Work out the finished part from the listing and answer in its coordinate system (mm). Face numbers are marked on the shaded views. A direction names the side the tool comes from. Round coordinates to 2 decimals unless told otherwise and drop trailing zeros. Loops run counter-clockwise (first coordinate to the right, second up) from the corner with the lowest first, then second, coordinate; pieces in that order, holes last. Notation, with made-up numbers: (82.25, 8) -> (100.25, 8) arc R19 ccw to (100.25, 40) -> close; hole circle Ø11 at (-38.75, 35). An arc over 180 degrees is marked (long way). Write item = value, one per line. Start each with the question number.
```python
from build123d import *

# Parameters (mm, degrees)
SKETCH_W        = 96
SKETCH_H        = 70
PAD_DEPTH       = 22.8
SKETCH001_W     = 92.6
SKETCH001_H     = 67
POCKET_DEPTH    = 21.8
SKETCH002_W     = 6.6
SKETCH002_H     = 6.6
PAD001_DEPTH    = 17.2
SKETCH003_W     = 61
SKETCH003_H     = 46
POCKET001_DEPTH = 1.001
SKETCH004_R     = 1.35
POCKET002_DEPTH = 10
SKETCH005_R     = 1.35
POCKET003_DEPTH = 10
SKETCH006_R     = 1.35
POCKET004_DEPTH = 10
SKETCH007_R     = 1.35
POCKET005_DEPTH = 10
POCKET006_DEPTH = 1.701
SKETCH009_W     = 7
SKETCH009_H     = 6.3
PAD002_DEPTH    = 12.2
SKETCH010_R     = 2.2
POCKET007_DEPTH = 13.201
SKETCH011_R     = 2.2
POCKET008_DEPTH = 13.201
SKETCH012_R     = 2.2
POCKET009_DEPTH = 13.201
SKETCH013_R     = 2.2
POCKET010_DEPTH = 13.201
SKETCH014_W     = 9.6
SKETCH014_H     = 15.6
POCKET011_DEPTH = 1.501
SKETCH015_W     = 8.6
SKETCH015_H     = 3.6
POCKET012_DEPTH = 1.501
FILLET_R        = 1
FILLET001_R     = 1
CHAMFER_SIZE    = 0.2
FILLET002_R     = 1
FILLET003_R     = 1


with BuildPart() as part:
    # Sketch → Pad (new body)
    with BuildSketch(Plane.XY):
        Rectangle(SKETCH_W, SKETCH_H)
    extrude(amount=PAD_DEPTH)

    # Sketch001 (on Face6 of Pad) → Pocket (cut)
    with BuildSketch(Plane.XY.offset(22.8)):
        Rectangle(SKETCH001_W, SKETCH001_H)
    extrude(amount=-POCKET_DEPTH, mode=Mode.SUBTRACT)

    # Sketch002 (on Face11 of Pocket) → Pad001 (join)
    with BuildSketch(Plane.XY.offset(1)):
        with Locations((-43, 30.2)):
            Rectangle(SKETCH002_W, SKETCH002_H)
        with Locations((43, 30.2)):
            Rectangle(SKETCH002_W, SKETCH002_H)
        with Locations((43, -30.2)):
            Rectangle(SKETCH002_W, SKETCH002_H)
        with Locations((-43, -30.2)):
            Rectangle(SKETCH002_W, SKETCH002_H)
    extrude(amount=PAD001_DEPTH)

    # Sketch003 (on Face13 of Pad001) → Pocket001 (cut, through all)
    with BuildSketch(Plane.XY.offset(1)):
        with Locations((0.3, 0.2)):
            Rectangle(SKETCH003_W, SKETCH003_H)
    extrude(amount=-POCKET001_DEPTH, mode=Mode.SUBTRACT)

    # Sketch004 (on Face19 of Pocket001) → Pocket002 (cut)
    with BuildSketch(Plane.XY.offset(18.2)):
        with Locations((-43, 30.2)):
            Circle(SKETCH004_R)
    extrude(amount=-POCKET002_DEPTH, mode=Mode.SUBTRACT)

    # Sketch005 (on Face16 of Pocket002) → Pocket003 (cut)
    with BuildSketch(Plane.XY.offset(18.2)):
        with Locations((43, 30.2)):
            Circle(SKETCH005_R)
    extrude(amount=-POCKET003_DEPTH, mode=Mode.SUBTRACT)

    # Sketch006 (on Face23 of Pocket003) → Pocket004 (cut)
    with BuildSketch(Plane.XY.offset(18.2)):
        with Locations((-43, -30.2)):
            Circle(SKETCH006_R)
    extrude(amount=-POCKET004_DEPTH, mode=Mode.SUBTRACT)

    # Sketch007 (on Face20 of Pocket004) → Pocket005 (cut)
    with BuildSketch(Plane.XY.offset(18.2)):
        with Locations((43, -30.2)):
            Circle(SKETCH007_R)
    extrude(amount=-POCKET005_DEPTH, mode=Mode.SUBTRACT)

    # Sketch008 (on Face14 of Pocket005) → Pocket006 (cut, through all)
    with BuildSketch(Plane.YZ.offset(-46.3)):
        with BuildLine():
            Line((-12.5, 22.8), (-6.5, 22.8))
            Line((-6.5, 22.8), (-6.5, 11.2))
            ThreePointArc((-12.5, 11.2), (-9.5, 8.2), (-6.5, 11.2))
            Line((-12.5, 11.2), (-12.5, 22.8))
        make_face()
        with BuildLine():
            Line((6.5, 22.8), (12.5, 22.8))
            Line((12.5, 22.8), (12.5, 11.2))
            ThreePointArc((6.5, 11.2), (9.5, 8.2), (12.5, 11.2))
            Line((6.5, 11.2), (6.5, 22.8))
        make_face()
    extrude(amount=-POCKET006_DEPTH, mode=Mode.SUBTRACT)

    # Sketch009 (on Face22 of Pocket006) → Pad002 (join)
    with BuildSketch(Plane.XY.offset(1)):
        with Locations((-29.7, -30.35)):
            Rectangle(SKETCH009_W, SKETCH009_H)
        with Locations((-14, -30.35)):
            Rectangle(SKETCH009_W, SKETCH009_H)
        with Locations((1.7, -30.35)):
            Rectangle(SKETCH009_W, SKETCH009_H)
        with Locations((17.4, -30.35)):
            Rectangle(SKETCH009_W, SKETCH009_H)
    extrude(amount=PAD002_DEPTH)

    # Sketch010 (on Face35 of Pad002) → Pocket007 (cut, through all)
    with BuildSketch(Plane.XY.offset(13.2)):
        with Locations((-29.7, -30.5)):
            Circle(SKETCH010_R)
    extrude(amount=-POCKET007_DEPTH, mode=Mode.SUBTRACT)

    # Sketch011 (on Face39 of Pocket007) → Pocket008 (cut, through all)
    with BuildSketch(Plane.XY.offset(13.2)):
        with Locations((-14, -30.5)):
            Circle(SKETCH011_R)
    extrude(amount=-POCKET008_DEPTH, mode=Mode.SUBTRACT)

    # Sketch012 (on Face43 of Pocket008) → Pocket009 (cut, through all)
    with BuildSketch(Plane.XY.offset(13.2)):
        with Locations((1.7, -30.5)):
            Circle(SKETCH012_R)
    extrude(amount=-POCKET009_DEPTH, mode=Mode.SUBTRACT)

    # Sketch013 (on Face47 of Pocket009) → Pocket010 (cut, through all)
    with BuildSketch(Plane.XY.offset(13.2)):
        with Locations((17.4, -30.5)):
            Circle(SKETCH013_R)
    extrude(amount=-POCKET010_DEPTH, mode=Mode.SUBTRACT)

    # Sketch014 (on Face23 of Pocket010) → Pocket011 (cut, through all)
    with BuildSketch(Plane.XZ.offset(-33.5)):
        with Locations((17.1, 15)):
            Rectangle(SKETCH014_W, SKETCH014_H)
    extrude(amount=-POCKET011_DEPTH, mode=Mode.SUBTRACT)

    # Sketch015 (on Face19 of Pocket011) → Pocket012 (cut, through all)
    with BuildSketch(Plane.XZ.offset(-33.5)):
        with Locations((30, 16.9)):
            Rectangle(SKETCH015_W, SKETCH015_H)
    extrude(amount=-POCKET012_DEPTH, mode=Mode.SUBTRACT)

    # Fillet
    fillet_edges = [part.edges().sort_by_distance(p)[0] for p in [
        (48, 35, 11.4),
        (-48, 35, 11.4),
        (-48, -35, 11.4),
        (48, -35, 11.4),
    ]]
    fillet(fillet_edges, radius=FILLET_R)

    # Fillet001
    fillet001_edges = [part.edges().sort_by_distance(p)[0] for p in [
        (-39.7, 26.9, 9.6),
        (39.7, 26.9, 9.6),
        (39.7, -26.9, 9.6),
        (20.9, -27.2, 7.1),
        (13.9, -27.2, 7.1),
        (5.2, -27.2, 7.1),
        (-1.8, -27.2, 7.1),
        (-10.5, -27.2, 7.1),
        (-17.5, -27.2, 7.1),
        (-26.2, -27.2, 7.1),
        (-33.2, -27.2, 7.1),
        (-39.7, -26.9, 9.6),
    ]]
    fillet(fillet001_edges, radius=FILLET001_R)

    # Chamfer
    chamfer_edges = [part.edges().sort_by_distance(p)[0] for p in [
        (15.2, -30.5, 0),
        (-0.5, -30.5, 0),
        (-16.2, -30.5, 0),
        (-31.9, -30.5, 0),
    ]]
    chamfer(chamfer_edges, length=CHAMFER_SIZE)

    # Fillet002
    fillet002_edges = [part.edges().sort_by_distance(p)[0] for p in [
        (34.3, 34.25, 15.1),
        (34.3, 34.25, 18.7),
        (25.7, 34.25, 18.7),
        (25.7, 34.25, 15.1),
    ]]
    fillet(fillet002_edges, radius=FILLET002_R)

    # Fillet003
    fillet003_edges = [part.edges().sort_by_distance(p)[0] for p in [
        (-30.2, 23.2, 0.5),
        (30.8, 23.2, 0.5),
        (30.8, -22.8, 0.5),
        (-30.2, -22.8, 0.5),
    ]]
    fillet(fillet003_edges, radius=FILLET003_R)


solid = part.part
```
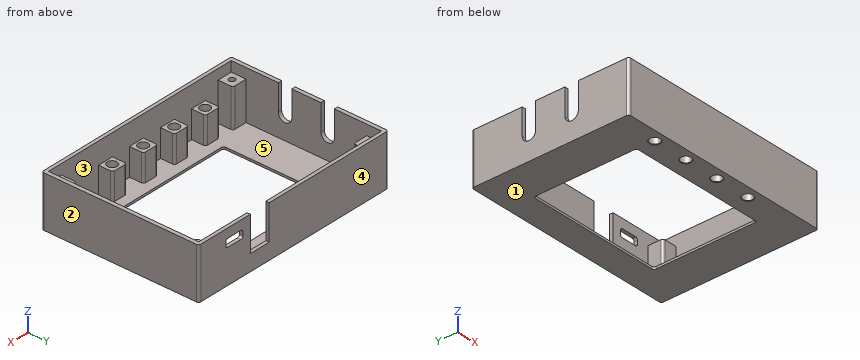
Item 1: Flat-ended cylindrical pins translate along their axes: pin 1 (2 mm diameter, centred on x = 42, y = 30, fed in from +Z); pin 2 (10 mm diameter, centred on x = 27, y = -27, fed in from +Z). Find the tip coordinate at first contact, or state that the pin passes through.
Item 2: Section B-B (z = 21) is taken. Determine the outline of the cut face in (x, y), then the cut area to 3 significant figures.
Item 3: A tool of negligible diameter and unlimited length cuts with its end or side. For the marked faces 4 and 5, from which of +Z, -Z, +X, -X, +Y, -Y can it reach the whole face along a straight path? Write none if from no direction.
Item 4: Section C-C (x = -43) is taken. Determine the outline of the cut face in (y, z), then the cut area to 3 significant figures.
Item 5: Section D-D (y = -9.5) is taken. Determine the outline of the cut face in (x, z), then the cut area to 3 significant figures.
Item 6: Section A-A (y = -2.5) is taken. Determine the outline of the cut face in (x, z), then the cut area to 3 significant figures.
Item 7: The mould has two halves that part along X. Classify the marked faces 1, 2 and 3: pulls with the +X half, pulls with the -X half, needs draft (parallel to the pull), parting line crosses it, or undercut.
Item 8: Find the intervals of material crossed by line 1 along Y through (x, z) = (43, 11.25); line 2 along Y through (x, z) = (41, 20.25); line 3 along X through (y, z) = (6.5, 9.25), in increasing order. Write a range as [from, to].
Worked answers:
q1.pin_1 = 18.2
q1.pin_2 = 1
q2.outline = (-48, -34) arc R1 ccw to (-47, -35) -> (47, -35) arc R1 ccw to (48, -34) -> (48, 34) arc R1 ccw to (47, 35) -> (21.9, 35) -> (21.9, 33.5) -> (46.3, 33.5) -> (46.3, -33.5) -> (-46.3, -33.5) -> (-46.3, -12.5) -> (-48, -12.5) -> close; (-48, -6.5) -> (-46.3, -6.5) -> (-46.3, 6.5) -> (-48, 6.5) -> close; (-48, 12.5) -> (-46.3, 12.5) -> (-46.3, 33.5) -> (12.3, 33.5) -> (12.3, 35) -> (-47, 35) arc R1 ccw to (-48, 34) -> close
q2.area = 480 mm2
q3.face_4 = +Z, -Z, +X, -X, +Y
q3.face_5 = +Z
q4.outline = (-35, 0) -> (35, 0) -> (35, 22.8) -> (33.5, 22.8) -> (33.5, 18.2) -> (31.55, 18.2) -> (31.55, 8.2) -> (28.85, 8.2) -> (28.85, 18.2) -> (26.9, 18.2) -> (26.9, 1) -> (-26.9, 1) -> (-26.9, 18.2) -> (-28.85, 18.2) -> (-28.85, 8.2) -> (-31.55, 8.2) -> (-31.55, 18.2) -> (-33.5, 18.2) -> (-33.5, 22.8) -> (-35, 22.8) -> close
q4.area = 308 mm2
q5.outline = (-48, 0) -> (-30.2, 0) -> (-30.2, 1) -> (-46.3, 1) -> (-46.3, 8.2) -> (-48, 8.2) -> close; (30.8, 0) -> (48, 0) -> (48, 22.8) -> (46.3, 22.8) -> (46.3, 1) -> (30.8, 1) -> close
q5.area = 84.3 mm2
q6.outline = (-48, 0) -> (-30.2, 0) -> (-30.2, 1) -> (-46.3, 1) -> (-46.3, 22.8) -> (-48, 22.8) -> close; (30.8, 0) -> (48, 0) -> (48, 22.8) -> (46.3, 22.8) -> (46.3, 1) -> (30.8, 1) -> close
q6.area = 109 mm2
q7.face_1 = needs draft
q7.face_2 = pulls with the +X half
q7.face_3 = undercut
q8.line_1 = [-35, -31.55], [-28.85, -26.9], [26.9, 28.85], [31.55, 35]
q8.line_2 = [-35, -33.5], [33.5, 35]
q8.line_3 = [-48, -46.3], [46.3, 48]
